Part model, mm, in its own coordinate system. A direction names the side the tool comes from. Give positions to 0.01 mm unless a question says otherwise; leave off trailing zeros. Order: outer loops, then holes, each group sorted by start corner. A loop starts at its lowest first (then second) coordinate and runs counter-clockwise, first axis right, second up. Notation, with made-up numbers: (-4.5, 27) -> (26.5, 27) arc R5 ccw to (26.5, 35) -> close; hole circle Ø3 at (-14, 62). An arc over 180 degrees is marked (long way). Write item = value, one per line. Start each with the question number.
Item 1: Band-saw the part on A-A on y = 66. Write the cut outline in (x, z), plus the area to 3 significant figures.
Item 2: Band-saw the part on B-B on x = 36.5. Write the cut outline in (y, z), plus the area to 3 significant figures.
Item 3: Pull direction X, two halves, no side cores. Call faces 4 (the face through (-117.5, 46, 3)), 5 (the face through (117.5, 46, 3)), 6 (the face through (56, 8.7, -108)), 7 (the face through (18.139, 29, -108)): +X half, -X half, draft (parallel to the pull), parting line (faces both ways), or undercut.
Item 4: Flat gauge pin, fed straight in: P1, Ø4, axis at x = -35, z = -58, coming from the +Y side. Where does the tip first touch, or does it go through?
Item 5: Band-saw the part on C-C on z = 97. Write the cut outline in (x, y).
Item 6: Tool access for faces 1 (the face through (9, 100, 118)), 2 (the face through (107.5, 49, 7)), 3 (the face through (56, 49.07, -108)): list every direction of +Z, -Z, +X, -X, +Y, -Y with a clear straight run to the whole face (end or side of a thin tool).
Item 7: Band-saw the part on D-D on y = 30.5. Write the cut outline in (x, z), plus the area to 3 significant figures.
Item 8: Drill centre lines: line 1 along X through (y, z) = (38, -88); line 2 along Z through (x, y) = (-92.5, 35); line 3 along Y through (x, z) = (2, -4.5). Where is each one in solid material? Low to high.
```python
from build123d import *

# Parameters (mm, degrees)
IZIM2_W                     = 215
IZIM2_H                     = 215
Y_KSEKLIK_EKSTR_ZYON1_DEPTH = 100
IZIM3_W                     = 235
IZIM3_H                     = 235
Y_KSEKLIK_EKSTR_ZYON2_DEPTH = 10
KES_EKSTR_ZYON1_REACH       = 283.125
IZIM5_W                     = 74.73555952
IZIM5_H                     = 40.37033127


with BuildPart() as part:
    # Çizim2 → Yükseklik-Ekstrüzyon1 (new body)
    with BuildSketch(Plane(origin=(0, 0, 0), x_dir=(1, 0, 0), z_dir=(0, 1, 0))):
        Polygon((117.5, 112.5), (117.5, 102.5), (117.5, -112.5), (117.5, -122.5), (107.5, -122.5), (-107.5, -122.5), (-117.5, -122.5), (-117.5, -112.5), (-117.5, 112.5), (-107.5, 112.5), (107.5, 112.5), align=None)
        with Locations((0, -5)):
            Rectangle(IZIM2_W, IZIM2_H, mode=Mode.SUBTRACT)
    extrude(amount=Y_KSEKLIK_EKSTR_ZYON1_DEPTH)

    # Çizim3 → Yükseklik-Ekstrüzyon2 (add)
    with BuildSketch(Plane.XZ):
        with Locations((0, 5)):
            Rectangle(IZIM3_W, IZIM3_H)
    extrude(amount=Y_KSEKLIK_EKSTR_ZYON2_DEPTH)

    # Çizim5 → Kes-Ekstrüzyon1 (cut, up to next)
    with BuildSketch(Plane(origin=(0, 0, -112.5), x_dir=(-1, 0, 0), z_dir=(0, 0, -1)), mode=Mode.PRIVATE) as kes_ekstr_zyon1_sk1:
        with Locations((-55.507242177, 28.884807523)):
            Rectangle(IZIM5_W, IZIM5_H)
    kes_ekstr_zyon1_tool1 = extrude(kes_ekstr_zyon1_sk1.sketch, amount=-KES_EKSTR_ZYON1_REACH, mode=Mode.PRIVATE) & part.part
    add(kes_ekstr_zyon1_tool1.solids().sort_by_distance((55.507242, 28.884808, -112.5))[0], mode=Mode.SUBTRACT)


solid = part.part
```
Values found:
q1.outline = (-117.5, -112.5) -> (117.5, -112.5) -> (117.5, 122.5) -> (-117.5, 122.5) -> close; hole (-107.5, -102.5) -> (107.5, -102.5) -> (107.5, 112.5) -> (-107.5, 112.5) -> close
q1.area = 9,000 mm^2
q2.outline = (-10, -112.5) -> (8.7, -112.5) -> (8.7, -102.5) -> (0, -102.5) -> (0, 112.5) -> (100, 112.5) -> (100, 122.5) -> (-10, 122.5) -> close; (49.07, -112.5) -> (100, -112.5) -> (100, -102.5) -> (49.07, -102.5) -> close
q2.area = 3,950 mm^2
q3.face_4 = -X half
q3.face_5 = +X half
q3.face_6 = undercut
q3.face_7 = undercut
q4.P1 = 0
q5.outline = (-117.5, -10) -> (117.5, -10) -> (117.5, 100) -> (107.5, 100) -> (107.5, 0) -> (-107.5, 0) -> (-107.5, 100) -> (-117.5, 100) -> close
q6.face_1 = +Z, -Z, +X, -X, +Y
q6.face_2 = +Y
q6.face_3 = -Z
q7.outline = (-117.5, -112.5) -> (18.14, -112.5) -> (18.14, -102.5) -> (-107.5, -102.5) -> (-107.5, 112.5) -> (107.5, 112.5) -> (107.5, -102.5) -> (92.88, -102.5) -> (92.88, -112.5) -> (117.5, -112.5) -> (117.5, 122.5) -> (-117.5, 122.5) -> close
q7.area = 8,250 mm^2
q8.line_1 = -117.5 to -107.5, 107.5 to 117.5
q8.line_2 = -112.5 to -102.5, 112.5 to 122.5
q8.line_3 = -10 to 0
